Can you work these out from the model? Positions are in its coordinate system, mm. A direction names the side the tool comes from. Coordinates: 2 decimals unless noted, no trailing zeros. Loops run counter-clockwise (first coordinate to the right, second up) from the corner with the lowest first, then second, coordinate; pieces in that order, holes last. Notation, with made-up numbers: (87, 12) -> (91, 12) arc R34 ccw to (91, 42) -> close; hole circle Ø5 at (70.25, -32). An arc over 180 degrees is marked (long way). Use one line per item in the form item = value. Start each with the question number.
(1) On a 3-axis mill with a long thin cutter (end or side, diameter ignored), from which of +Z, -Z, +X, -X, +Y, -Y can I reach the whole of each face in a straight line? I mean faces 1 (the cylindrical face through (4.484, 2.17, 0.53)), 2 (the flat face through (6.75, 0, 5)), 3 (the flat face through (6.913, -0.028, 36.528)). Say none if no direction works.
(2) Imagine slicing it at D-D (y = 4). List the corners of the cut face in (x, z) for me, plus the area to 3 significant figures.
(3) Thinking about a two-plate mould opening in X: for faces 4 (the flat face through (6, 2, 19)), 5 (the cylindrical face through (-0.338, 2.578, 0.493)), 6 (the cylindrical face through (7.125, -1.549, 39.465)), which applies, released by +X, released by -X, zero draft, split by the parting line, or undercut?
(4) I'm going to push flat-ended pins straight in: pin 1 (1 mm diameter, centred on x = -3.5, y = 0, fed in from +Z); pin 2 (2.5 mm diameter, centred on x = 5.5, z = 17, fed in from -Y); pin 3 (1 mm diameter, centred on x = 6.5, z = 28.5, fed in from +Y); pin 4 (3 mm diameter, centred on y = 0, z = 31, fed in from +X). Where does each tip first touch, or does it pass through?
(5) I need wall thicknesses on line 1 (Y direction, x = 0, z = 0.2); line 2 (X direction, y = 0, z = 0.3); line 3 (Z direction, x = -1.75, y = 2). Which ranges of each line are inside material? Lowest first, please. Write a range as [from, to].
(6) Imagine slicing it at B-B (x = 0). List the corners of the cut face in (y, z) for me, plus the area to 3 significant figures.
(7) Imagine slicing it at C-C (z = 31). List the corners of the cut face in (x, y) for me.
(8) Imagine slicing it at A-A (y = 0). List the corners of the cut face in (x, z) for me.
```python
from build123d import *

# Parameters (mm, degrees)
F0_R     = 2.6
F1_DEPTH = 40
F3_DEPTH = 12.5
F4_R     = 1.5


with BuildPart() as f1:
    # F0 (on Top) → F1 (new body)
    with BuildSketch(Plane.XY):
        with BuildLine():
            Line((8.75, 2), (4.3084219849, 2))
            ThreePointArc((4.3084219849, 2), (-4.75, 0), (4.3084219849, -2))
            Line((4.3084219849, -2), (8.75, -2))
            Line((8.75, -2), (8.75, 2))
        make_face()
        Circle(F0_R, mode=Mode.SUBTRACT)
    extrude(amount=F1_DEPTH)

    # F2 (on Front) → F3 (cut, symmetric)
    with BuildSketch(Plane.XZ):
        with BuildLine():
            Line((10.2479401976, 42.5026379526), (7.7201425001, 39.757464375))
            Line((7.7201425001, 39.757464375), (6.082376492, 33.2064003424))
            ThreePointArc((6.082376492, 33.2064003424), (5.5603768051, 29.9093586064), (5.6234510612, 26.5718461314))
            Line((5.6234510612, 26.5718461314), (7.75, 6.7463273263))
            Line((7.75, 6.7463273263), (7.75, 3))
            ThreePointArc((7.75, 3), (6.8713203436, 0.8786796564), (4.75, 0))
            Line((4.75, 0), (-9.0971523896, 0))
            Line((-9.0971523896, 0), (-9.0971523896, -6.0571944341))
            Line((-9.0971523896, -6.0571944341), (12.3898674946, -5.0901651477))
            Line((12.3898674946, -5.0901651477), (10.2479401976, 42.5026379526))
        make_face()
        with BuildLine():
            Line((-9.0971523896, 1), (4.75, 1))
            ThreePointArc((4.75, 1), (6.1642135624, 1.5857864376), (6.75, 3))
            Line((6.75, 3), (6.75, 6.6928490996))
            Line((6.75, 6.6928490996), (4.629154591, 26.4651946927))
            ThreePointArc((4.629154591, 26.4651946927), (4.5627606372, 29.978365719), (5.1122339919, 33.4489359674))
            Line((5.1122339919, 33.4489359674), (6.75, 40))
            Line((6.75, 40), (-4.4842101634, 43.9101681113))
            Line((-4.4842101634, 43.9101681113), (-11.3513292745, 32.9360663891))
            Line((-11.3513292745, 32.9360663891), (-9.0971523896, 1))
        make_face()
        Polygon((5.6231939234, 43.9101681113), (6.75, 40), (7.7201425001, 39.757464375), (10.2479401976, 42.5026379526), align=None)
    extrude(amount=F3_DEPTH, both=True, mode=Mode.SUBTRACT)

    # F4 (call 1 of 4: OpenCascade refuses the feature's edges together)
    f4_edges = [f1.edges().sort_by_distance(p)[0] for p in [
        (7.235071, -2, 39.878732),
    ]]
    fillet(f4_edges, radius=F4_R)

    # F4#2 (call 2 of 4)
    f4_2_edges = [f1.edges().sort_by_distance(p)[0] for p in [
        (7.235071, 2, 39.878732),
    ]]
    fillet(f4_2_edges, radius=F4_R)

    # F4#3 (call 3 of 4)
    f4_3_edges = [f1.edges().sort_by_distance(p)[0] for p in [
        (4.308422, -2, 0.5),
    ]]
    fillet(f4_3_edges, radius=F4_R)

    # F4#4 (call 4 of 4)
    f4_4_edges = [f1.edges().sort_by_distance(p)[0] for p in [
        (4.308422, 2, 0.5),
    ]]
    fillet(f4_4_edges, radius=F4_R)


solid = f1.part
```
Worked out:
q1.face_1 = +Z, -Z, +X, +Y
q1.face_2 = -X, +Y, -Y
q1.face_3 = +X, +Y, -Y
q2.outline = (-2.56, 0) -> (2.56, 0) -> (2.56, 1) -> (-2.56, 1) -> close
q2.area = 5.12 mm2
q3.face_4 = zero draft
q3.face_5 = undercut
q3.face_6 = released by +X
q4.pin_1 = 1
q4.pin_2 = -2
q4.pin_3 = through
q4.pin_4 = 5.92
q5.line_1 = [-4.75, -2.6], [2.6, 4.75]
q5.line_2 = [-4.75, -2.6], [2.6, 6.06]
q5.line_3 = [0, 1]
q6.outline = (-4.75, 0) -> (-2.6, 0) -> (-2.6, 1) -> (-4.75, 1) -> close; (2.6, 0) -> (4.75, 0) -> (4.75, 1) -> (2.6, 1) -> close
q6.area = 4.30 mm2
q7.outline = (4.66, -2) -> (5.67, -2) -> (5.67, 2) -> (4.66, 2) -> close
q8.outline = (-4.75, 0) -> (-2.6, 0) -> (-2.6, 1) -> (-4.75, 1) -> close; (2.6, 0) -> (4.75, 0) arc R3 ccw to (7.75, 3) -> (7.75, 6.75) -> (5.62, 26.57) arc R19 cw to (6.08, 33.21) -> (7.72, 39.76) -> (6.75, 40) -> (5.11, 33.45) arc R20 ccw to (4.63, 26.47) -> (6.75, 6.69) -> (6.75, 3) arc R2 cw to (4.75, 1) -> (2.6, 1) -> close
